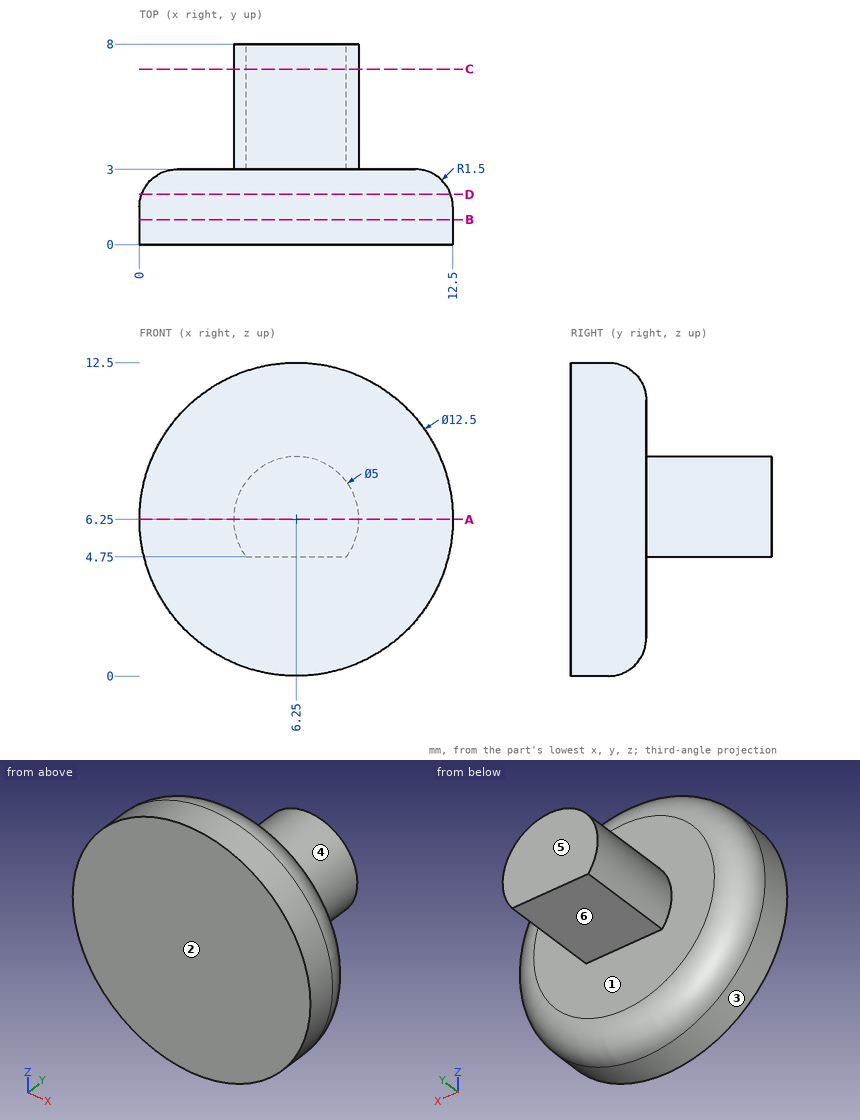
Source: three-view drawing plus pictorial views. Frame: mm from the lowest corner of the part. A direction names the side the tool comes from. Round coordinates to 2 decimals unless told otherwise and drop trailing zeros. Loops run counter-clockwise (first coordinate to the right, second up) from the corner with the lowest first, then second, coordinate; pieces in that order, holes last. Notation, with made-up numbers: (78, -9.75) -> (104, -9.75) arc R17 cw to (104, 6.25) -> close; hole circle Ø6 at (27, 56). An arc over 180 degrees is marked (long way). Use one line per item in the form item = value.
Item 1: Cut plane C-C on y = 7. Output: boundary loops of the cut face in (x, z).
Evaluation:
outline = (4.25, 4.75) -> (8.25, 4.75) arc R2.5 ccw (long way) to start
Item 2: Cut plane A-A on z = 6.25. Output: boundary loops of the cut face in (x, y), then the cut area to 3 significant figures.
Evaluation:
outline = (0, 0) -> (12.5, 0) -> (12.5, 1.5) arc R1.5 ccw to (11, 3) -> (8.75, 3) -> (8.75, 8) -> (3.75, 8) -> (3.75, 3) -> (1.5, 3) arc R1.5 ccw to (0, 1.5) -> close
area = 61.5 mm2
Item 3: Contact query for flat-ended pins moving along their axis: pin 1 Ø4.5 at (x, y) = (6.5, 4.5) entering from -Z; pin 2 Ø1 at (x, y) = (3.5, 2) entering from -Z. Output: stop coordinate, or through.
Evaluation:
pin_1 = 0.2
pin_2 = 0.47
Item 4: Material intervals for probe 1 along Y at (x, z) = (5.5, 4.25); probe 2 along Z at (x, y) = (8.75, 2); probe 3 along Z at (x, y) = (9.5, 2.5), sorted ascending.
Evaluation:
probe_1 = 0 to 3
probe_2 = 0.62 to 11.88
probe_3 = 1.36 to 11.14
Item 5: Cut plane D-D on y = 2. Output: boundary loops of the cut face in (x, z).
Evaluation:
outline = circle Ø12.33 at (6.25, 6.25)
Item 6: Access query for the marked faces 4, 5 and 6. Directions: +Z, -Z, +X, -X, +Y, -Y. A direction counts if a zero-diameter tool reaches every point of the face in a straight line with its end or side. Return the directions, or none.
Evaluation:
face_4 = +Y
face_5 = +Z, -Z, +X, -X, +Y
face_6 = -Z, +X, -X, +Y
Item 7: Cut plane B-B on y = 1. Output: boundary loops of the cut face in (x, z).
Evaluation:
outline = circle Ø12.5 at (6.25, 6.25)
Item 8: Draft query along Y for the marked faces 1, 2 and 3. Return one class per face: released by +Y, released by -Y, zero draft, split by the parting line, or undercut.
Evaluation:
face_1 = released by +Y
face_2 = released by -Y
face_3 = zero draft
